Build history of the part. All positions in model axes, mm. A direction names the side the tool comes from. Give positions to 0.01 mm unless a question says otherwise; leave off trailing zeros. Order: outer loops, then holes, each group sorted by start corner. A loop starts at its lowest first (then second) coordinate and runs counter-clockwise, first axis right, second up. Notation, with made-up numbers: (55.25, 89.25) -> (88.25, 89.25) arc R24 ccw to (88.25, 110.25) -> close; hole circle Ø7 at (56, 76.25). An arc over 180 degrees is marked (long way). One line per item, written item: value. Start each with the question number.
(1) Which spindle directions (+Z, -Z, +X, -X, +Y, -Y) get a long thin tool onto all of the face, cutting with end or side? Do faces 1 (the flat face through (76, 10, 13.5)), 2 (the flat face through (85, 28, -1)), 3 (the flat face through (39.5, 5, 3)), 4 (the flat face through (69.9, 29, 7)). Say none if no direction does.
(2) Probe line 1 (Y direction, x = 71.5, z = 4.25); line 2 (Y direction, x = 61.5, z = -0.7); line 3 (Z direction, x = 61, y = 20). List the from-to ranges inside material, lowest first.
(3) Saw through at B-B on x = 74.5. Give the cut face in (y, z).
(4) Saw through at D-D on x = 62. Give the cut face in (y, z).
(5) Two-plate mould, pull along X, no slides. Class faces 5 (the flat face through (86, 47, 0)), 6 (the cylindrical face through (3.32, 53.89, -0.79)), 7 (the cylindrical face through (84.14, 55.1, -0.79)): +X half, -X half, draft (parallel to the pull), parting line (faces both ways), or undercut.
(6) Saw through at A-A on z = 8.5. Give the cut face in (x, y).
(7) Saw through at C-C on y = 44. Give the cut face in (x, z), plus the area to 3 significant figures.
(8) Pin check, flat tips, straight feed: pin 1 (6.5 mm diameter, centred on y = 7, z = 2, fed in from -X); pin 2 (1.3 mm diameter, centred on y = 19.5, z = -1, fed in from +X); pin 3 (1.7 mm diameter, centred on x = 86, y = 10, fed in from -Z); pin 4 (4 mm diameter, centred on y = 12, z = 5.5, fed in from -X). Stop position of each tip, or through.
```python
from build123d import *

# Parameters (mm, degrees)
F0_R      = 1.4
F1_DEPTH  = 1.6
F3_DEPTH  = 13.5
F4_W      = 15.1002969221
F4_H      = 13.1
F4_W_2    = 2.1
F5_DEPTH  = 14.8
F6_W      = 6
F6_H      = 15
F7_DEPTH  = 5.5
F9_DEPTH  = 2.5
F10_W     = 15
F10_H     = 11
F11_DEPTH = 6
F12_W     = 7.5
F12_H     = 6
F13_DEPTH = 2.5


with BuildPart() as f1:
    # F0 (on Top) → F1 (new body)
    with BuildSketch(Plane.XY):
        with BuildLine():
            ThreePointArc((0, 3), (0.8786796564, 0.8786796564), (3, 0))
            Line((3, 0), (82, 0))
            ThreePointArc((82, 0), (84.1213203436, 0.8786796564), (85, 3))
            Line((85, 3), (85, 53))
            ThreePointArc((85, 53), (84.1213203436, 55.1213203436), (82, 56))
            Line((82, 56), (3, 56))
            ThreePointArc((3, 56), (0.8786796564, 55.1213203436), (0, 53))
            Line((0, 53), (0, 3))
        make_face()
        with Locations((3.5, 3.5)):
            Circle(F0_R, mode=Mode.SUBTRACT)
        with Locations((61.5, 3.5)):
            Circle(F0_R, mode=Mode.SUBTRACT)
        with Locations((3.5, 52.5)):
            Circle(F0_R, mode=Mode.SUBTRACT)
        with Locations((61.5, 52.5)):
            Circle(F0_R, mode=Mode.SUBTRACT)
    extrude(amount=-F1_DEPTH)

    # F2 (on face) → F3 (join)
    with BuildSketch(Plane.XY):
        with BuildLine():
            Line((84.9171904292, 2.3), (87.1, 2.3))
            Line((87.1, 2.3), (87.1, 18.2))
            Line((87.1, 18.2), (85, 18.2))
            Line((85, 18.2), (85, 3))
            ThreePointArc((85, 3), (84.9792256786, 2.6475594288), (84.9171904292, 2.3))
        make_face()
        with BuildLine():
            Line((65, 2.3), (84.9171904292, 2.3))
            ThreePointArc((84.9171904292, 2.3), (84.9792256786, 2.6475594288), (85, 3))
            Line((85, 3), (85, 18.2))
            Line((85, 18.2), (65, 18.2))
            Line((65, 18.2), (65, 2.3))
        make_face()
    extrude(amount=F3_DEPTH)

    # F4 (on face) → F5 (join)
    with BuildSketch(Plane.XY):
        with Locations((77.4498515389, 28.95)):
            Rectangle(F4_W, F4_H)
        with BuildLine():
            Line((84.9580398915, 53.5), (69.8997030779, 53.5))
            Line((69.8997030779, 53.5), (69.8997030779, 40.4))
            Line((69.8997030779, 40.4), (85, 40.4))
            Line((85, 40.4), (85, 53))
            ThreePointArc((85, 53), (84.9894915684, 53.2508787808), (84.9580398915, 53.5))
        make_face()
        with BuildLine():
            Line((87.1, 53.5), (84.9580398915, 53.5))
            ThreePointArc((84.9580398915, 53.5), (84.9894915684, 53.2508787808), (85, 53))
            Line((85, 53), (85, 40.4))
            Line((85, 40.4), (87.1, 40.4))
            Line((87.1, 40.4), (87.1, 53.5))
        make_face()
        with Locations((86.05, 28.95)):
            Rectangle(F4_W_2, F4_H)
    extrude(amount=F5_DEPTH)

    # F6 (on face) → F7 (join)
    with BuildSketch(Plane.XY):
        with Locations((53.5, 7.5)):
            Rectangle(F6_W, F6_H)
    extrude(amount=F7_DEPTH)

    # F8 (on face) → F9 (join)
    with BuildSketch(Plane.XZ):
        with BuildLine():
            Line((55.3428853505, 1.0606884287), (51.6571146495, 4.4393115713))
            ThreePointArc((51.6571146495, 4.4393115713), (51.8106884287, 0.9071146495), (55.3428853505, 1.0606884287))
        make_face()
        with BuildLine():
            ThreePointArc((56, 2.75), (54.4063075151, 5.0799370567), (51.6571146495, 4.4393115713))
            Line((51.6571146495, 4.4393115713), (55.3428853505, 1.0606884287))
            ThreePointArc((55.3428853505, 1.0606884287), (55.8299370567, 1.8436924849), (56, 2.75))
        make_face()
    extrude(amount=F9_DEPTH)

    # F10 (on face) → F11 (join)
    with BuildSketch(Plane.XY):
        with Locations((32, 5.5)):
            Rectangle(F10_W, F10_H)
    extrude(amount=F11_DEPTH)

    # F12 (on face) → F13 (join)
    with BuildSketch(Plane.XY):
        with Locations((10.55, 3)):
            Rectangle(F12_W, F12_H)
    extrude(amount=F13_DEPTH)


solid = f1.part
```
Results below:
1. face 1: +Z, +X, -X, -Y
1. face 2: -Z, +X, +Y, -Y
1. face 3: +Z, +Y, -Y
1. face 4: +Z, -X, +Y
2. line 1: y = 2.3 to 18.2, 22.4 to 35.5, 40.4 to 53.5
2. line 2: y = 0 to 2.1, 4.9 to 51.1, 53.9 to 56
2. line 3: z = -1.6 to 0
3. outline: (0, -1.6) -> (56, -1.6) -> (56, 0) -> (53.5, 0) -> (53.5, 14.8) -> (40.4, 14.8) -> (40.4, 0) -> (35.5, 0) -> (35.5, 14.8) -> (22.4, 14.8) -> (22.4, 0) -> (18.2, 0) -> (18.2, 13.5) -> (2.3, 13.5) -> (2.3, 0) -> (0, 0) -> close
4. outline: (0, -1.6) -> (2.19, -1.6) -> (2.19, 0) -> (0, 0) -> close; (4.81, -1.6) -> (51.19, -1.6) -> (51.19, 0) -> (4.81, 0) -> close; (53.81, -1.6) -> (56, -1.6) -> (56, 0) -> (53.81, 0) -> close
5. face 5: draft
5. face 6: undercut
5. face 7: +X half
6. outline: (65, 2.3) -> (87.1, 2.3) -> (87.1, 18.2) -> (65, 18.2) -> close; (69.9, 22.4) -> (87.1, 22.4) -> (87.1, 35.5) -> (69.9, 35.5) -> close; (69.9, 40.4) -> (87.1, 40.4) -> (87.1, 53.5) -> (69.9, 53.5) -> close
7. outline: (0, -1.6) -> (85, -1.6) -> (85, 0) -> (87.1, 0) -> (87.1, 14.8) -> (69.9, 14.8) -> (69.9, 0) -> (0, 0) -> close
7. area: 391 mm²
8. pin 1: stops at x = 0
8. pin 2: stops at x = 85
8. pin 3: stops at z = 0
8. pin 4: stops at x = 24.5
